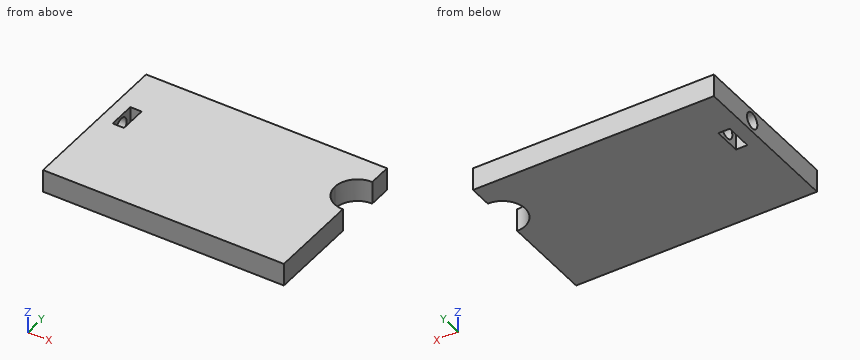
```python
from build123d import *

# Parameters (mm, degrees)
F0_W     = 3
F0_H     = 10
F0_H_2   = 3
F1_DEPTH = 5
F2_R     = 1.75
F3_DEPTH = 20
F4_DEPTH = 20


# Not quite as in the source:
# - a feature names something its author has since deleted; it is built from what else it names


with BuildPart() as f1:
    # F0 (on Top) → F1 (new body)
    with BuildSketch(Plane.XY):
        with BuildLine():
            Line((-5, 25), (-47.5, 25))
            Line((-47.5, 25), (-47.5, 22))
            Line((-47.5, 22), (-47.5, 19))
            Line((-47.5, 19), (-50, 19))
            Line((-50, 19), (-50, 0))
            Line((-50, 0), (0, 0))
            Line((0, 0), (0, 20))
            ThreePointArc((0, 20), (-3.5355339059, 21.4644660941), (-5, 25))
        make_face()
        Polygon((-50, 22), (-53, 22), (-53, 0), (-50, 0), (-50, 19), align=None)
        with Locations((-51.5, 30)):
            Rectangle(F0_W, F0_H)
        with Locations((-51.5, 23.5)):
            Rectangle(F0_W, F0_H_2)
        with BuildLine():
            Line((0, 35), (-50, 35))
            Line((-50, 35), (-50, 25))
            Line((-50, 25), (-47.5, 25))
            Line((-47.5, 25), (-5, 25))
            ThreePointArc((-5, 25), (-3.5355339059, 28.5355339059), (0, 30))
            Line((0, 30), (0, 35))
        make_face()
    extrude(amount=F1_DEPTH)

    # F2 (on face) → F3 (cut)
    with BuildSketch(Plane(origin=(-53, 0, 0), x_dir=(0, -1, 0), z_dir=(-1, 0, 0))):
        with Locations((-22, 2.5274456161)):
            Circle(F2_R)
    extrude(amount=-F3_DEPTH, mode=Mode.SUBTRACT)

    # F2 (on face) → F4 (cut)
    with BuildSketch(Plane(origin=(-53, 0, 0), x_dir=(0, -1, 0), z_dir=(-1, 0, 0))):
        with BuildLine():
            ThreePointArc((22, 4.2774456161), (20.25, 2.5274456161), (22, 0.7774456161))
            Line((22, 0.7774456161), (22, 2.5274456161))
            Line((22, 2.5274456161), (22, 4.2774456161))
        make_face()
        with BuildLine():
            ThreePointArc((22, 0.7774456161), (23.2361299407, 1.2887032015), (23.7499961, 2.5237510221))
            Line((23.7499961, 2.5237510221), (22, 2.5274456161))
            Line((22, 2.5274456161), (22, 0.7774456161))
        make_face()
        with BuildLine():
            Line((22, 2.5274456161), (23.7499961, 2.5237510221))
            ThreePointArc((23.7499961, 2.5237510221), (23.749999025, 2.5255983181), (23.75, 2.5274456161))
            ThreePointArc((23.75, 2.5274456161), (23.2374368671, 3.7648824831), (22, 4.2774456161))
            Line((22, 4.2774456161), (22, 2.5274456161))
        make_face()
    extrude(amount=-F4_DEPTH, mode=Mode.SUBTRACT)


solid = f1.part
```
Input: part model. Units: mm. Frame: model coordinates. Coordinates: 2 decimals unless noted, no trailing zeros. Loops run counter-clockwise (first coordinate to the right, second up) from the corner with the lowest first, then second, coordinate; pieces in that order, holes last.
Q1. Section B-B, the plane x = -48.5. Return the cut outline in (y, z).
Results are:
outline: (0, 0) - (19, 0) - (19, 5) - (0, 5) - close; (25, 0) - (35, 0) - (35, 5) - (25, 5) - close
Q2. Section A-A, the plane y = 22. Return the cut outline in (x, z), and give its area (3 significant figures).
Results are:
outline: (-53, 0) - (-50, 0) - (-50, 0.78) - (-53, 0.78) - close; (-53, 4.28) - (-50, 4.28) - (-50, 5) - (-53, 5) - close; (-47.5, 0) - (-4, 0) - (-4, 5) - (-47.5, 5) - (-47.5, 4.28) - (-33, 4.28) - (-33, 0.78) - (-47.5, 0.78) - close
area: 171 mm2
Q3. Section C-C, the plane z = 1.95. Return the cut outline in (x, y).
Results are:
outline: (-53, 0) - (0, 0) - (0, 20) arc R5 cw to (0, 30) - (0, 35) - (-53, 35) - (-53, 23.65) - (-50, 23.65) - (-50, 25) - (-47.5, 25) - (-47.5, 23.65) - (-33, 23.65) - (-33, 20.35) - (-47.5, 20.35) - (-47.5, 19) - (-50, 19) - (-50, 20.35) - (-53, 20.35) - close
Q4. Line query: line 1 along Z through (x, y) = (-52.1, 22); line 2 along Y through (x, z) = (-49, 1.55); line 3 along Y through (x, z) = (-41.5, 2.65). Output: solid intervals per line, ascending.
Results are:
line 1: z = 0 to 0.78, 4.28 to 5
line 2: y = 0 to 19, 25 to 35
line 3: y = 0 to 20.25, 23.75 to 35
Q5. Section D-D, the plane x = -38. Return the cut outline in (y, z).
Results are:
outline: (0, 0) - (35, 0) - (35, 5) - (0, 5) - close; hole circle Ø3.5 at (22, 2.53)
Q6. Contact query for flat-ended pins moving along their axis: pin 1 (3 mm diameter, centred on y = 21.5, z = 2, fed in from -X); pin 2 (2 mm diameter, centred on y = 24.5, z = 3.5, fed in from +X); pin 3 (3 mm diameter, centred on y = 22, z = 2.53, fed in from -X). Output: stop coordinate, or through.
Results are:
pin 1: stops at x = -53
pin 2: stops at x = -4.77
pin 3: stops at x = -33
